Here's the drawing with two shaded views (mm, measured from the low corner). I have some questions. Give positions to 0.01 mm unless a question says otherwise; leave off trailing zeros. Write each loop counter-clockwise with the first axis right and the second up, starting at its lowest first coordinate (ties: lowest second). Pieces come first, ordered by that corner, then holes. Notation, with made-up numbers: (36, -38) -> (86, -38) arc R16 ccw to (86, -10) -> close; hole circle Ø1 at (12, -28). An arc over 180 degrees is marked (long way). One line per item, written item: value.
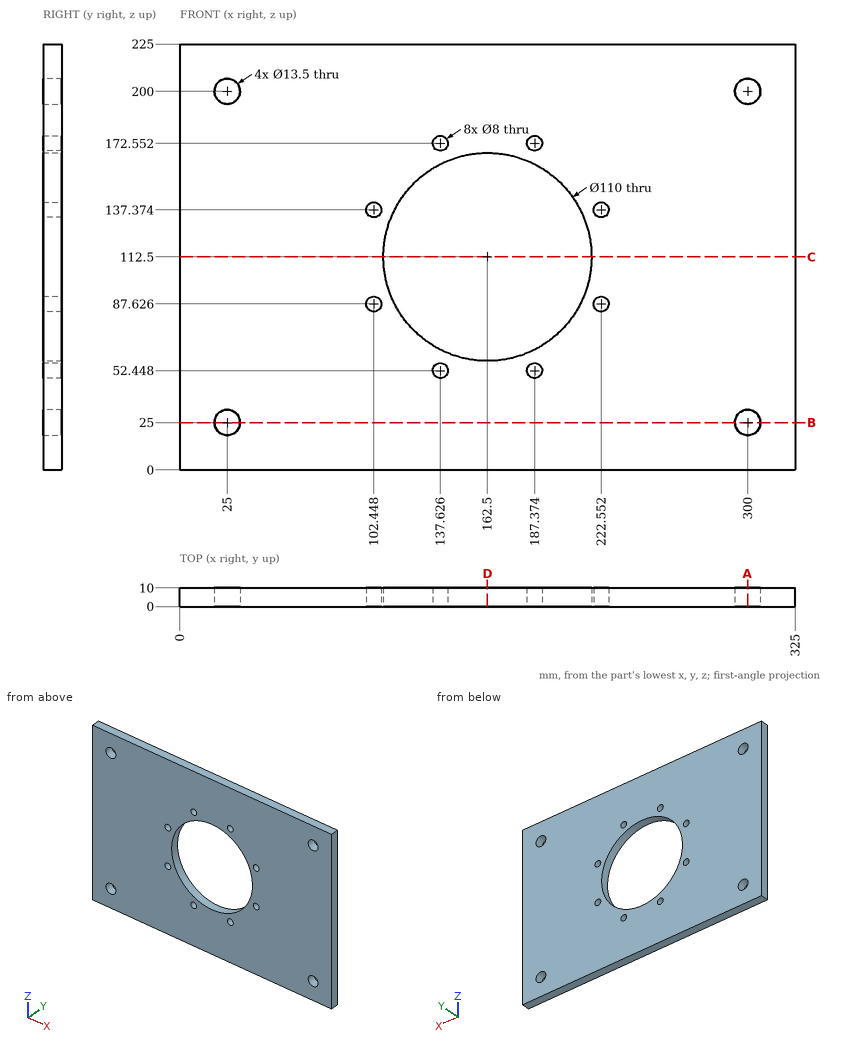
1) If we section it at C-C (z = 112.5): Write out the boundary of the cut face in (x, y).
Answer list:
outline: (0, 0) -> (107.5, 0) -> (107.5, 10) -> (0, 10) -> close; (217.5, 0) -> (325, 0) -> (325, 10) -> (217.5, 10) -> close
2) I need wall thicknesses on L1, parallel to Z at x = 25, y = 6; L2, parallel to X at y = 8, z = 200; L3, parallel to Z at x = 23.5, y = 8. Which ranges of each line are inside material? Lowest first, please.
Answer list:
L1: z = 0 to 18.25, 31.75 to 193.25, 206.75 to 225
L2: x = 0 to 18.25, 31.75 to 293.25, 306.75 to 325
L3: z = 0 to 18.42, 31.58 to 193.42, 206.58 to 225
3) If we section it at A-A (x = 300): Write out the boundary of the cut face in (y, z), and give its area (3 significant figures).
Answer list:
outline: (0, 0) -> (10, 0) -> (10, 18.25) -> (0, 18.25) -> close; (0, 31.75) -> (10, 31.75) -> (10, 193.25) -> (0, 193.25) -> close; (0, 206.75) -> (10, 206.75) -> (10, 225) -> (0, 225) -> close
area: 1,980 mm^2
4) If we section it at D-D (x = 162.5): Write out the boundary of the cut face in (y, z).
Answer list:
outline: (0, 0) -> (10, 0) -> (10, 57.5) -> (0, 57.5) -> close; (0, 167.5) -> (10, 167.5) -> (10, 225) -> (0, 225) -> close
5) If we section it at B-B (z = 25): Write out the boundary of the cut face in (x, y), and give its area (3 significant figures).
Answer list:
outline: (0, 0) -> (18.25, 0) -> (18.25, 10) -> (0, 10) -> close; (31.75, 0) -> (293.25, 0) -> (293.25, 10) -> (31.75, 10) -> close; (306.75, 0) -> (325, 0) -> (325, 10) -> (306.75, 10) -> close
area: 2,980 mm^2
